Can you work these out from the drawing? Everything is in mm from the part's minimum corner. A direction names the side the tool comes from. Round coordinates to 2 decimals unless told otherwise and drop trailing zeros. Order: outer loops, then holes, each group sorted by start corner. A loop starts at its lowest first (then second) coordinate and runs counter-clockwise, first axis right, second up. Notation, with made-up numbers: (17, 62) - (62, 62) arc R12 cw to (62, 85) - close; hole circle Ø7 at (-21.75, 2.25). An arc over 180 degrees is marked (long way). Write item = value, one per line.
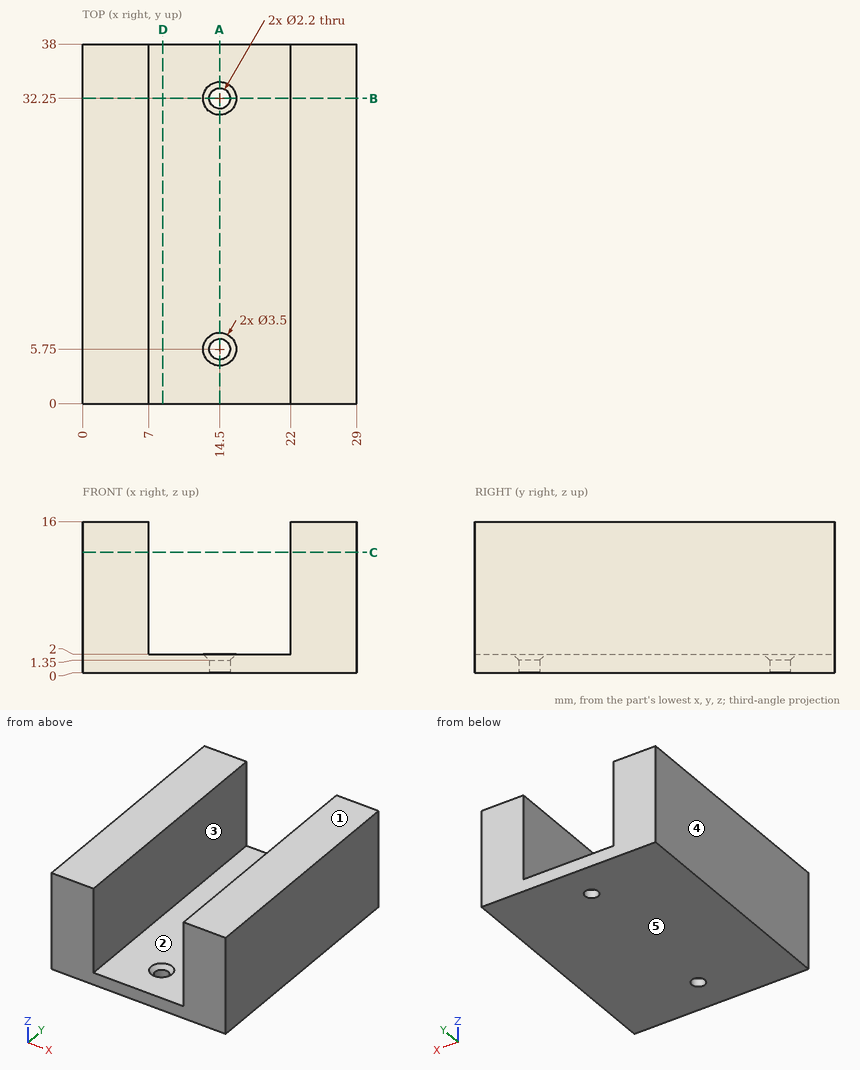
(1) On a 3-axis mill with a long thin cutter (end or side, diameter ignored), from which of +Z, -Z, +X, -X, +Y, -Y can I reach the whole of each face in a straight line? I mean the marked faces 1 and 2. Say none if no direction works.
Computed:
face_1 = +Z, +X, -X, +Y, -Y
face_2 = +Z, +Y, -Y
(2) Thinking about a two-plate mould opening in X: for the marked faces 3, 4 and 5, which applies, +X half, -X half, draft (parallel to the pull), parting line (faces both ways), or undercut?
Computed:
face_3 = undercut
face_4 = -X half
face_5 = draft
(3) If I drill on line 1 (Y direction, x = 14.5, z = 0.55); line 2 (X direction, y = 32.25, z = 0.35); line 3 (X direction, y = 22, z = 14), over which ranges is the centre line in solid material (lowest first)? Write a range as from..to.
Computed:
line_1 = 0..4.65, 6.85..31.15, 33.35..38
line_2 = 0..13.4, 15.6..29
line_3 = 0..7, 22..29
(4) If we section it at D-D (x = 8.5): Write out the boundary of the cut face in (y, z), plus the area to 3 significant figures.
Computed:
outline = (0, 0) - (38, 0) - (38, 2) - (0, 2) - close
area = 76.0 mm^2
(5) If we section it at B-B (y = 32.25): Write out the boundary of the cut face in (x, z), plus the area to 3 significant figures.
Computed:
outline = (0, 0) - (13.4, 0) - (13.4, 1.35) - (12.75, 2) - (7, 2) - (7, 16) - (0, 16) - close; (15.6, 0) - (29, 0) - (29, 16) - (22, 16) - (22, 2) - (16.25, 2) - (15.6, 1.35) - close
area = 249 mm^2
(6) If we section it at C-C (z = 12.75): Write out the boundary of the cut face in (x, y), plus the area to 3 significant figures.
Computed:
outline = (0, 0) - (7, 0) - (7, 38) - (0, 38) - close; (22, 0) - (29, 0) - (29, 38) - (22, 38) - close
area = 532 mm^2
(7) If we section it at A-A (x = 14.5): Write out the boundary of the cut face in (y, z), plus the area to 3 significant figures.
Computed:
outline = (0, 0) - (4.65, 0) - (4.65, 1.35) - (4, 2) - (0, 2) - close; (6.85, 0) - (31.15, 0) - (31.15, 1.35) - (30.5, 2) - (7.5, 2) - (6.85, 1.35) - close; (33.35, 0) - (38, 0) - (38, 2) - (34, 2) - (33.35, 1.35) - close
area = 66.4 mm^2
(8) Will these pins go through, and if not, where does the flat tip stop? P1, Ø8, axis at x = 13, z = 14, coming from the +Y side; P2, Ø1, axis at y = 25.5, z = 9, coming from the -X side; P3, Ø4.5, axis at x = 12, y = 16, coming from the +Z side.
Computed:
P1 = through
P2 = 0
P3 = 2
